Study the drawing (mm; zero at the part's minimum x, y, z) and answer. Coordinates: 2 decimals unless noted, no trailing zeros. Order: outer loops, then holes, each group sorted by start corner. A loop starts at its lowest first (then second) coordinate and runs counter-clockwise, first axis right, second up.
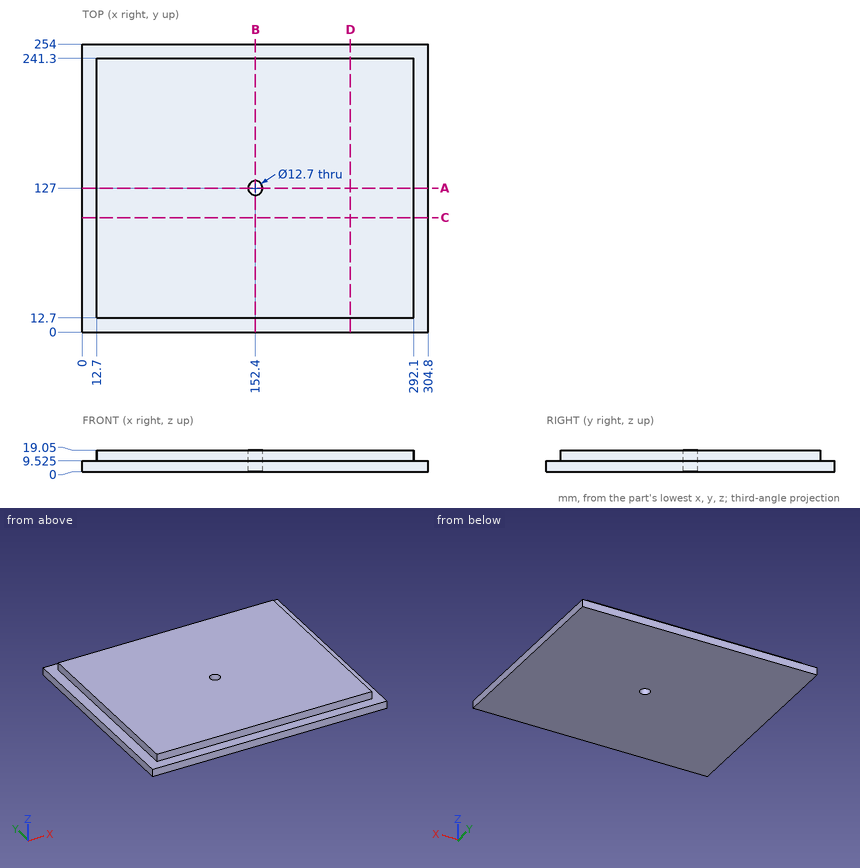
(1) Find section B-B on x = 152.4. Determine the outline of the cut face in (y, z) (3 decimals), then the cut area to 3 significant figures.
(2) Find section D-D on x = 236. Determine the outline of the cut face in (y, z) (3 decimals), then the cut area to 3 significant figures.
(3) Given pin 1 Ø7.5 at (x, y) = (152.4, 127) entering from -Z; pin 2 Ø2 at (y, z) = (51.5, 12) entering from +X; pin 3 Ø5 at (x, z) = (97, 16) entering from +Y; pin 4 Ø3 at (x, z) = (133.5, 13) entering from -Y, each flat-ended and moving along its own axis, determine where each tip first touches the part or whether it passes through.
(4) Find section C-C on y = 101. Determine the outline of the cut face in (x, z) (3 decimals).
(5) Find the intervals of material crossed by probe 1 along Y at (x, z) = (152.4, 7.5); probe 2 along Y at (x, z) = (152.4, 13.5); probe 3 along Y at (x, z) = (159, 12), in increasing order.
(6) Find section A-A on y = 127. Determine the outline of the cut face in (x, z) (3 decimals).
Resolved:
1. outline: (0, 0) - (120.65, 0) - (120.65, 19.05) - (12.7, 19.05) - (12.7, 9.525) - (0, 9.525) - close; (133.35, 0) - (254, 0) - (254, 9.525) - (241.3, 9.525) - (241.3, 19.05) - (133.35, 19.05) - close
1. area: 4,350 mm2
2. outline: (0, 0) - (254, 0) - (254, 9.525) - (241.3, 9.525) - (241.3, 19.05) - (12.7, 19.05) - (12.7, 9.525) - (0, 9.525) - close
2. area: 4,600 mm2
3. pin 1: passes through
3. pin 2: stops at x = 292.1
3. pin 3: stops at y = 241.3
3. pin 4: stops at y = 12.7
4. outline: (0, 0) - (304.8, 0) - (304.8, 9.525) - (292.1, 9.525) - (292.1, 19.05) - (12.7, 19.05) - (12.7, 9.525) - (0, 9.525) - close
5. probe 1: y = 0 to 120.65, 133.35 to 254
5. probe 2: y = 12.7 to 120.65, 133.35 to 241.3
5. probe 3: y = 12.7 to 241.3
6. outline: (0, 0) - (146.05, 0) - (146.05, 19.05) - (12.7, 19.05) - (12.7, 9.525) - (0, 9.525) - close; (158.75, 0) - (304.8, 0) - (304.8, 9.525) - (292.1, 9.525) - (292.1, 19.05) - (158.75, 19.05) - close
